Read the model definition and answer for the solid it produces. Units are mm, in the model's axes. Face numbers are marked on the shaded views. Round coordinates to 2 decimals unless told otherwise and drop trailing zeros. Order: outer loops, then holes, each group sorted by start corner. A loop starts at its lowest first (then second) coordinate and runs counter-clockwise, first axis right, second up. Notation, with made-up numbers: (42, -38) -> (83, -38) arc R32 ccw to (83, -2) -> close; hole circle Ø5 at (59.5, -37.5). An arc over 180 degrees is marked (long way). Answer as a JSON object with one key per item and string values. Group by question number.
Item 1: The mould has two halves that part along X. Classify the marked faces 1, 2, 3 and 4: pulls with the +X half, pulls with the -X half, needs draft (parallel to the pull), parting line crosses it, or undercut.
Item 2: Section A-A, the plane x = 37.5 is taken. Write down the section's boundary in (y, z), plus the area to 3 significant figures.
Item 3: Consider probe 1 along Y at (x, z) = (0, 5); probe 2 along X at (y, z) = (-42, 11.5); probe 3 along X at (y, z) = (-38.5, 8.25). Determine where each line is inside the solid, lowest interval first. Write a range as from..to.
Item 4: Section D-D, the plane x = -77 is taken. Write down the section's boundary in (y, z).
Item 5: Section C-C, the plane z = 3.25 is taken. Count the separate pieces of the cut face and the enclosed holes in it, plus the area to 3 significant figures.
Item 6: Section B-B, the plane y = 50.5 is taken. Write down the section's boundary in (x, z).
Item 7: Given P1, Ø6, axis at y = -83, z = 3.5, coming from the -X side; P2, Ø3, axis at x = 11.5, z = 10.5, coming from the -Y side; P3, Ø2, axis at y = -66, z = 4.5, coming from the +X side; P4, Ø12.5, axis at x = 63.06, y = -36.41, coming from the +Z side (3 decimals), each flat-ended and moving along its own axis, determine where each tip first touches the part or whether it passes through.
from build123d import *

# Parameters (mm, degrees)
F0_R     = 10.31875
F0_R_2   = 57.15
F1_DEPTH = 12.7


with BuildPart() as f1:
    # F0 (on Top) → F1 (new body)
    with BuildSketch(Plane.XY):
        with BuildLine():
            ThreePointArc((1.587462, -114.288976), (81.381622, -80.25909), (114.3, 0))
            ThreePointArc((114.3, 0), (110.608097, 28.8156), (99.770887, 55.769706))
            ThreePointArc((99.770887, 55.769706), (97.611888, 56.35625), (98.183425, 58.51927))
            ThreePointArc((98.183425, 58.51927), (0, 114.3), (-98.183425, 58.51927))
            ThreePointArc((-98.183425, 58.51927), (-97.609141, 57.938972), (-97.399204, 57.15))
            ThreePointArc((-97.399204, 57.15), (-98.188185, 55.777949), (-99.770887, 55.769706))
            ThreePointArc((-99.770887, 55.769706), (-98.986704, -57.15), (-1.587462, -114.288976))
            ThreePointArc((-1.587462, -114.288976), (0, -112.7125), (1.587462, -114.288976))
        make_face()
        with Locations((-63.05647, -36.40567)):
            Circle(F0_R, mode=Mode.SUBTRACT)
        with Locations((63.05647, -36.40567)):
            Circle(F0_R, mode=Mode.SUBTRACT)
        Circle(F0_R_2, mode=Mode.SUBTRACT)
        with Locations((0, 72.8091)):
            Circle(F0_R, mode=Mode.SUBTRACT)
    extrude(amount=F1_DEPTH)


solid = f1.part
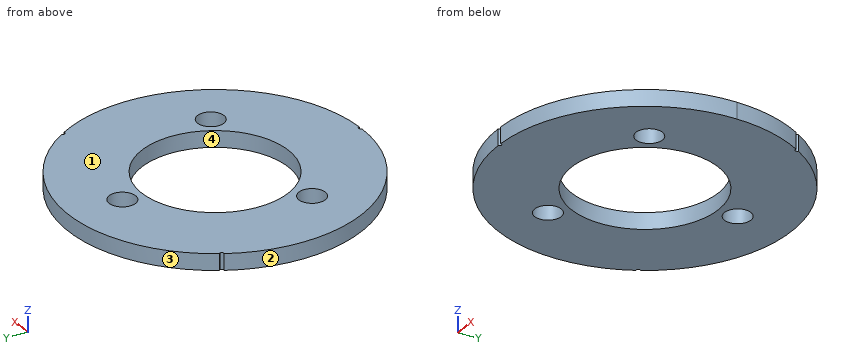
Values found:
{
 "1": {"face 1": "needs draft", "face 2": "pulls with the -X half", "face 3": "parting line crosses it", "face 4": "undercut"},
 "2": {"outline": "(-107.97, 0) -> (-43.13, 0) -> (-43.13, 12.7) -> (-107.97, 12.7) -> close; (43.13, 0) -> (107.97, 0) -> (107.97, 12.7) -> (43.13, 12.7) -> close", "area": "1,650 mm2"},
 "3": {"probe 1": "-112.71..-57.15, 57.15..62.49, 83.13..114.3", "probe 2": "-106.3..-71.73, -54.39..-38.76, 38.76..54.39, 71.73..106.3", "probe 3": "-107.62..-73.16, -52.95..-42.24, 42.24..52.95, 73.16..107.62"},
 "4": {"outline": "(-84.47, 0) -> (84.47, 0) -> (84.47, 12.7) -> (-84.47, 12.7) -> close"},
 "5": {"separate pieces": "1", "enclosed holes": "4", "area": "29,800 mm2"},
 "6": {"outline": "(-102.54, 0) -> (-26.76, 0) -> (-26.76, 12.7) -> (-102.54, 12.7) -> close; (26.76, 0) -> (102.54, 0) -> (102.54, 12.7) -> (26.76, 12.7) -> close"},
 "7": {"P1": "x = -81.64", "P2": "y = -113.86", "P3": "x = 94.02", "P4": "through"}
}
